from build123d import *

# Parameters (mm, degrees)
SKETCH1_R           = 17.5
BOSS_EXTRUDE1_DEPTH = 6.86
SKETCH2_R           = 12.5
CUT_EXTRUDE1_DEPTH  = 6.86
SKETCH3_R           = 1.25
CUT_EXTRUDE2_DEPTH  = 6.86
CIRPATTERN2_COUNT   = 6


with BuildPart() as part:
    # Sketch1 → Boss-Extrude1 (new body)
    with BuildSketch(Plane(origin=(0, 0, 0), x_dir=(1, 0, 0), z_dir=(0, 1, 0))):
        Circle(SKETCH1_R)
    extrude(amount=BOSS_EXTRUDE1_DEPTH)

    # Sketch2 → Cut-Extrude1 (cut)
    with BuildSketch(Plane(origin=(0, 6.86, 0), x_dir=(1, 0, 0), z_dir=(0, 1, 0))):
        Circle(SKETCH2_R)
    extrude(amount=-CUT_EXTRUDE1_DEPTH, mode=Mode.SUBTRACT)

    # Sketch3 → Cut-Extrude2 (cut)
    with BuildSketch(Plane(origin=(0, 6.86, 0), x_dir=(1, 0, 0), z_dir=(0, 1, 0))):
        with Locations((0, 15)):
            Circle(SKETCH3_R)
    cut_extrude2 = extrude(amount=-CUT_EXTRUDE2_DEPTH, mode=Mode.SUBTRACT)

    # CirPattern2: Cut-Extrude2 ×6 about axis
    cirpattern2_axis = Axis((0, 0, 0), (0, 1, 0))
    for i in range(1, CIRPATTERN2_COUNT):
        add(cut_extrude2.rotate(cirpattern2_axis, i * 360 / CIRPATTERN2_COUNT), mode=Mode.SUBTRACT)


solid = part.part
For this review, take the finished solid that the model builds, in its own axes (mm). Give positions to 0.01 mm unless a question says otherwise; leave off trailing zeros. Loops run counter-clockwise (first coordinate to the right, second up) from the corner with the lowest first, then second, coordinate; pieces in that order, holes last. Notation, with made-up numbers: M 14,-13 L 50,-13 A22 ccw 50,-1 Z; hole C -3.75,40.5 d3. An arc over 180 degrees is marked long. Answer as a JSON object with one key per item and string values. Group by question number.
Q1. For probe 1 along Z at (x, y) = (0, 5.25); probe 2 along X at (y, z) = (3, -8.5); probe 3 along Z at (x, y) = (14, 6.5), list the stretches that pass through material, from the lowest coordinate up. Write a range as [from, to].
Q2. Add section D-D on y = 5.25. Give the boundary of the cut face in (x, z), and give its area (3 significant figures).
Q3. Add section B-B on x = 0. Give the boundary of the cut face in (y, z), and give its area (3 significant figures).
Q4. Add section A-A on z = 0. Give the boundary of the cut face in (x, y).
Q5. Insertion check: P1, Ø4, axis at y = 2, z = -8.5, coming from the +X side; P2, Ø1.5, axis at y = 4.5, z = 5.5, coming from the -X side. Each pin has a flat end and moves straight along its axis. Give the tip position at first contact, or say it passes through.
Q6. Mouldability with a two-part tool opening along X and no side actions: class faces 1 (the cylindrical face through (-13.662, 3.478, -6.446)), 2 (the flat face through (-5, 6.86, 12)), 3 (the cylindrical face through (14.145, 3.478, 7.979)), 4 (the cylindrical face through (-13.887, 3.382, 10.648)) as +X half, -X half, draft (parallel to the pull), parting line (faces both ways), or undercut.
Q7. Add section C-C on x = -9.5. Give the boundary of the cut face in (y, z), and give its area (3 significant figures).
Checked values:
{
 "1": {"probe 1": "[-17.5, -16.25], [-13.75, -12.5], [12.5, 13.75], [16.25, 17.5]", "probe 2": "[-15.3, -13.74], [-12.24, -9.17], [9.17, 12.24], [13.74, 15.3]", "probe 3": "[-10.5, -8.24], [-6.76, 6.76], [8.24, 10.5]"},
 "2": {"outline": "C 0,0 d35; hole C -12.99,-7.5 d2.5; hole C -12.99,7.5 d2.5; hole C 0,0 d25; hole C 0,-15 d2.5; hole C 0,15 d2.5; hole C 12.99,-7.5 d2.5; hole C 12.99,7.5 d2.5", "area": "442 mm²"},
 "3": {"outline": "M 0,-17.5 L 6.86,-17.5 L 6.86,-16.25 L 0,-16.25 Z; M 0,-13.75 L 6.86,-13.75 L 6.86,-12.5 L 0,-12.5 Z; M 0,12.5 L 6.86,12.5 L 6.86,13.75 L 0,13.75 Z; M 0,16.25 L 6.86,16.25 L 6.86,17.5 L 0,17.5 Z", "area": "34.3 mm²"},
 "4": {"outline": "M -17.5,0 L -12.5,0 L -12.5,6.86 L -17.5,6.86 Z; M 12.5,0 L 17.5,0 L 17.5,6.86 L 12.5,6.86 Z"},
 "5": {"P1": "x = 16.25", "P2": "x = -16.84"},
 "6": {"face 1": "undercut", "face 2": "draft", "face 3": "undercut", "face 4": "parting line"},
 "7": {"outline": "M 0,-14.7 L 6.86,-14.7 L 6.86,-8.12 L 0,-8.12 Z; M 0,8.12 L 6.86,8.12 L 6.86,14.7 L 0,14.7 Z", "area": "90.2 mm²"}
}
